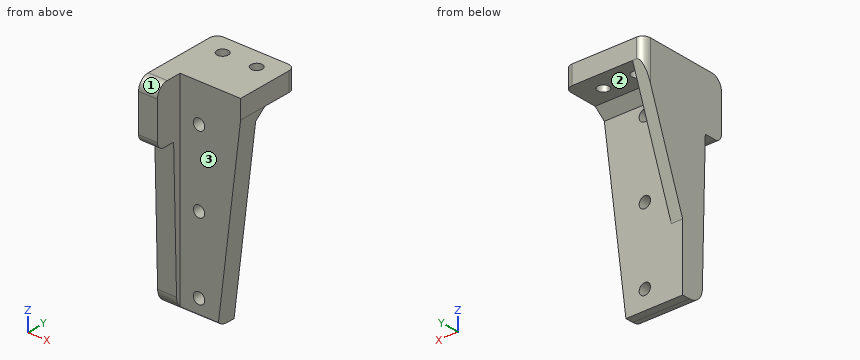
```python
from build123d import *

# Parameters (mm, degrees)
SKETCH_1_W          = 15
SKETCH_1_H          = 50
EXTRUDE_1_DEPTH     = 5
SKETCH_3_W          = 50
SKETCH_3_H          = 1
SKETCH_3_W_2        = 10
SKETCH_3_H_2        = 5
EXTRUDE_2_DEPTH     = 5
FILLET_1_R          = 4
FILLET_2_R          = 2
SKETCH_4_R          = 1.5
CUT_EXTRUDE_1_DEPTH = 5
SKETCH_5_R          = 1.5
EXTRUDE_3_DEPTH     = 5
CHAMFER_1_SIZE      = 2.5
FILLET_4_R          = 3
EXTRUDE_4_DEPTH     = 3
FILLET_5_R          = 2


with BuildPart() as part:
    # 草图1 → 凸台-拉伸1 (new body)
    with BuildSketch(Plane(origin=(0, 0, 0), x_dir=(1, 0, 0), z_dir=(0, 1, 0))):
        Rectangle(SKETCH_1_W, SKETCH_1_H)
        Polygon((7.5, -25), (13.5, -25), (7.5, 25), align=None)
    extrude(amount=EXTRUDE_1_DEPTH)

    # 草图3 → 凸台-拉伸2 (add)
    with BuildSketch(Plane.ZY.offset(7.5)):
        with Locations((0, -0.5)):
            Rectangle(SKETCH_3_W, SKETCH_3_H)
        Polygon((15, -2), (25, -2), (25, -1), (-25, -1), align=None)
        with Locations((20, -4.5)):
            Rectangle(SKETCH_3_W_2, SKETCH_3_H_2)
    extrude(amount=-EXTRUDE_2_DEPTH)

    # 圆角1
    fillet_1_edges = [part.edges().sort_by_distance(p)[0] for p in [
        (-5, -1, -25),
    ]]
    fillet(fillet_1_edges, radius=FILLET_1_R)

    # 圆角2
    fillet_2_edges = [part.edges().sort_by_distance(p)[0] for p in [
        (-5, -7, 15),
    ]]
    fillet(fillet_2_edges, radius=FILLET_2_R)

    # 草图4 → 切除-拉伸1 (cut)
    with BuildSketch(Plane.XZ):
        with Locations(Location((2.5, 20, 0), (0, 0, 270))):
            Circle(SKETCH_4_R)
        with Locations(Location((2.5, 0, 0), (0, 0, 270))):
            Circle(SKETCH_4_R)
        with Locations(Location((2.5, -20, 0), (0, 0, 270))):
            Circle(SKETCH_4_R)
    extrude(amount=-CUT_EXTRUDE_1_DEPTH, mode=Mode.SUBTRACT)

    # 草图5 → 凸台-拉伸3 (add)
    with BuildSketch(Plane.XY.offset(25)):
        Polygon((13.5, 5), (13.5, 0), (-2.5, 0), (-2.5, -7), (-7.5, -7), (-7.5, 5), (-7.5, 17), (13.5, 17), align=None)
        with Locations((-1.5, 12)):
            Circle(SKETCH_5_R, mode=Mode.SUBTRACT)
        with Locations((7.5, 12)):
            Circle(SKETCH_5_R, mode=Mode.SUBTRACT)
    extrude(amount=EXTRUDE_3_DEPTH)

    # 倒角1
    chamfer_1_edges = [part.edges().sort_by_distance(p)[0] for p in [
        (3, 5, 25),
    ]]
    chamfer(chamfer_1_edges, length=CHAMFER_1_SIZE)

    # 圆角4
    fillet_4_edges = [part.edges().sort_by_distance(p)[0] for p in [
        (-5, -7, 30),
    ]]
    fillet(fillet_4_edges, radius=FILLET_4_R)

    # 草图6 → 凸台-拉伸4 (add)
    with BuildSketch(Plane.ZY.offset(7.5)):
        Polygon((25, 17), (25, 7.5), (22.5, 5), (-7.5, 5), align=None)
    extrude(amount=-EXTRUDE_4_DEPTH)

    # 圆角5
    fillet_5_edges = [part.edges().sort_by_distance(p)[0] for p in [
        (13.5, 17, 27.5),
        (-7.5, 17, 27.5),
    ]]
    fillet(fillet_5_edges, radius=FILLET_5_R)


solid = part.part
```
Geometry check sheet. Reference: the model listing, model coordinates, mm. Face numbers are marked on the shaded views. A direction names the side the tool comes from. Coordinates: 2 decimals unless noted, no trailing zeros. Write each loop counter-clockwise with the first axis right and the second up, starting at its lowest first coordinate (ties: lowest second). Pieces come first, ordered by that corner, then holes. Notation, with made-up numbers: M 49.25,-19.75 L 70.25,-19.75 A12 ccw 70.25,3.25 Z; hole C 66,10 d6. An arc over 180 degrees is marked long. One line per item, written item: value. Start each with the question number.
(1) Sectioned sample at C-C, the plane x = -1. Enter the section's corners in (y, z), and give its area (3 significant figures).
(2) Scan lines: line 1 along Y through (x, z) = (7.5, 28.8); line 2 along X through (y, z) = (1.25, 0); line 3 along Y through (x, z) = (0.25, 26). Record each from-to range of solid material in increasing order. Write a range as [from, to].
(3) Depth check by flat-ended pin: pin 1 (1.5 mm diameter, centred on y = 6.5, z = 12, fed in from +X); pin 2 (12 mm diameter, centred on x = 1, z = -0.5, fed in from -Y); pin 3 (2.5 mm diameter, centred on x = 2.5, z = 0, fed in from -Y) (3 decimals); pin 4 (8 mm diameter, centred on x = -2.5, z = 5, fed in from -Y). Enter the tip coordinate at first touch or a pass-through.
(4) Sectioned sample at D-D, the plane z = 14. Enter the section's corners in (x, y) (3 decimals).
(5) Sectioned sample at B-B, the plane z = -20. Enter the section's corners in (x, y) (3 decimals), and give its area (3 significant figures).
(6) Tool access check on the marked faces 1, 2 and 3. Record the directions out of +Z, -Z, +X, -X, +Y, -Y that give a thin tool (end or side, any length) a straight path to the whole face; none if there is none.
(7) Sectioned sample at A-A, the plane y = 12. Enter the section's corners in (x, z).
Filled sheet:
1. outline: M 0,-23.75 A4 ccw 2.9,-25 L 5,-25 L 5,22.5 L 7.5,25 L 10.59,25 L 10.59,30 L 0,30 Z; M 13.41,25 L 17,25 L 17,30 L 13.41,30 Z
1. area: 323 mm²
2. line 1: [0, 10.5], [13.5, 17]
2. line 2: [-7.5, 1], [4, 10.5]
2. line 3: [0, 17]
3. pin 1: x = -4.5
3. pin 2: y = -1.73
3. pin 3: through
3. pin 4: y = -1.85
4. outline: M -7.5,-1.975 L -2.5,-1.975 L -2.5,0 L 12.18,0 L 12.18,5 L -4.5,5 L -4.5,12.938 L -7.5,12.938 Z
5. outline: M -7.5,-1.125 L -2.5,-1.125 L -2.5,0 L 1,0 L 1,5 L -7.5,5 Z; M 4,0 L 8.1,0 L 8.1,5 L 4,5 Z
5. area: 68.6 mm²
6. face 1: +Z, +X, -X, -Y
6. face 2: -Z, +X, +Y
6. face 3: +Z, -Z, +X, -Y
7. outline: M -7.5,11.46 L -4.5,11.46 L -4.5,25 L -3,25 L -3,30 L -7.5,30 Z; M 0,25 L 6,25 L 6,30 L 0,30 Z; M 9,25 L 13.5,25 L 13.5,30 L 9,30 Z
